Geometry check sheet. Reference: drawing and pictorial views, mm from the part's lowest x, y, z. A direction names the side the tool comes from. Give positions to 0.01 mm unless a question says otherwise; leave off trailing zeros. Write each loop counter-clockwise with the first axis right and the second up, starting at its lowest first coordinate (ties: lowest second). Pieces come first, ordered by that corner, then holes. Notation, with made-up numbers: (85.5, 32.25) - (127.5, 32.25) arc R6 cw to (127.5, 37.25) - close; hole circle Ø4 at (20, 20.5). An arc over 180 degrees is marked (long way). Put each result on its own line as item: value.
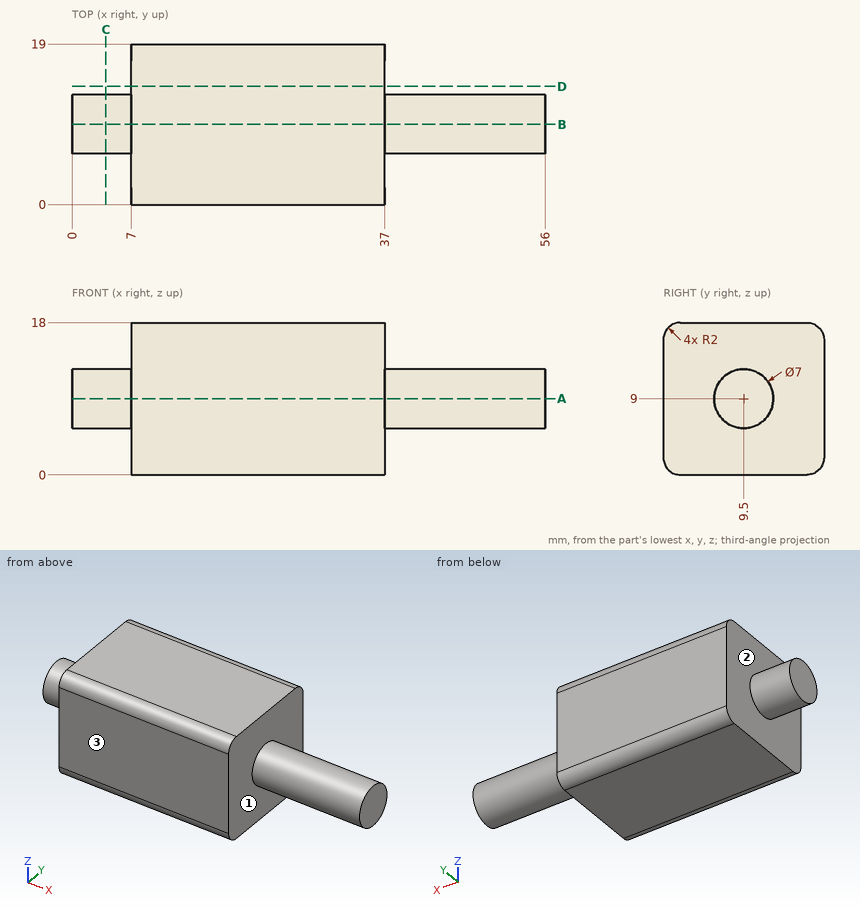
Q1. Section check B-B, the plane y = 9.5. Record the cut outline in (x, z), plus the area to 3 significant figures.
Answers follow:
outline: (0, 5.5) - (7, 5.5) - (7, 0) - (37, 0) - (37, 5.5) - (56, 5.5) - (56, 12.5) - (37, 12.5) - (37, 18) - (7, 18) - (7, 12.5) - (0, 12.5) - close
area: 722 mm2
Q2. Go/stop test with flat-tipped pins: pin 1 Ø1 at (y, z) = (12.5, 15.5) entering from -X; pin 2 Ø5 at (x, z) = (47.5, 6.5) entering from +Y; pin 3 Ø5 at (x, z) = (48.5, 11.5) entering from -Y. Record where each tip stops, or that it passes through.
Answers follow:
pin 1: stops at x = 7
pin 2: stops at y = 13
pin 3: stops at y = 6
Q3. Section check D-D, the plane y = 14. Record the cut outline in (x, z).
Answers follow:
outline: (7, 0) - (37, 0) - (37, 18) - (7, 18) - close
Q4. Section check A-A, the plane z = 9. Record the cut outline in (x, y), plus the area to 3 significant figures.
Answers follow:
outline: (0, 6) - (7, 6) - (7, 0) - (37, 0) - (37, 6) - (56, 6) - (56, 13) - (37, 13) - (37, 19) - (7, 19) - (7, 13) - (0, 13) - close
area: 752 mm2
Q5. Scan lines: line 1 along X through (y, z) = (3, 10); line 2 along Y through (x, z) = (52.5, 9); line 3 along Z through (x, y) = (42.5, 10.25). Record each from-to range of solid material in increasing order.
Answers follow:
line 1: x = 7 to 37
line 2: y = 6 to 13
line 3: z = 5.58 to 12.42
Q6. Set-up check for the marked faces 1, 2 and 3: record each of +Z, -Z, +X, -X, +Y, -Y from which the full face is reachable in a straight line by a thin tool's end or side.
Answers follow:
face 1: +X
face 2: -X
face 3: +Z, -Z, +X, -X, -Y
Q7. Section check C-C, the plane x = 4. Record the cut outline in (y, z), plus the area to 3 significant figures.
Answers follow:
outline: circle Ø7 at (9.5, 9)
area: 38.5 mm2
